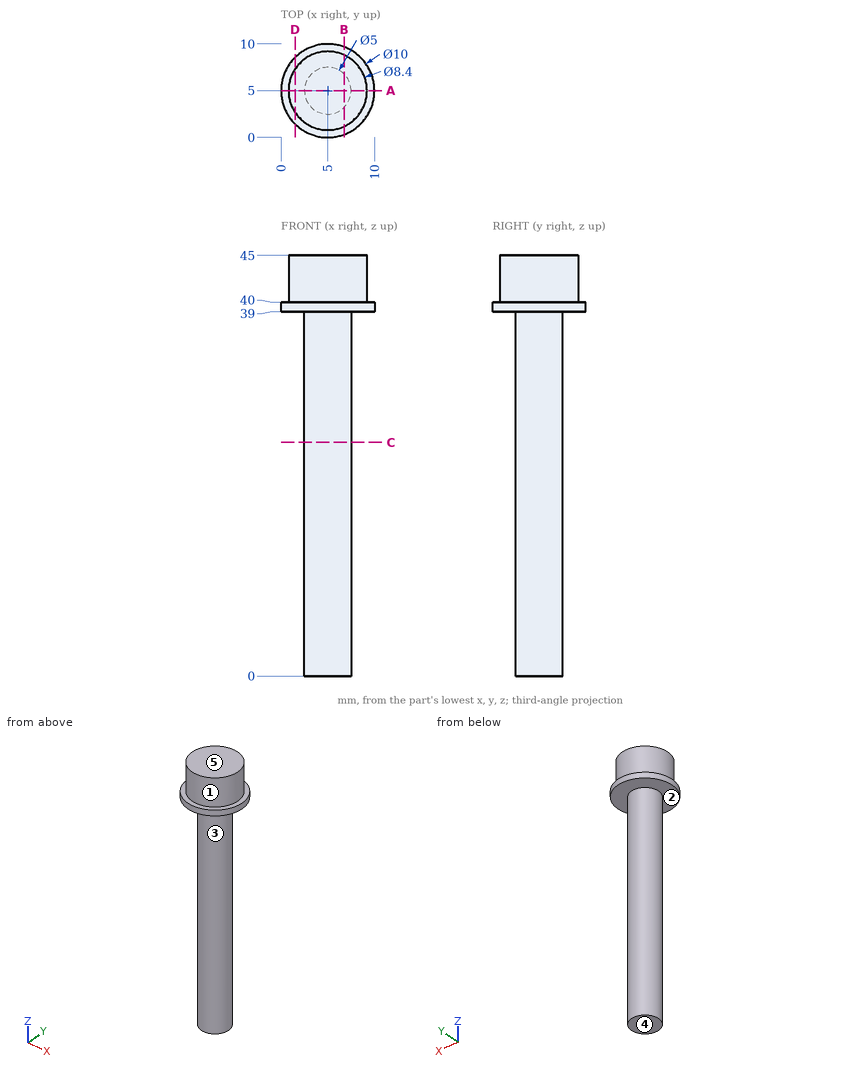
Here's the drawing with two shaded views (mm, measured from the low corner). I have some questions. A direction names the side the tool comes from. Round coordinates to 2 decimals unless told otherwise and drop trailing zeros. Order: outer loops, then holes, each group sorted by start corner. A loop starts at its lowest first (then second) coordinate and runs counter-clockwise, first axis right, second up. Notation, with made-up numbers: (15.25, 24.5) -> (51.25, 24.5) arc R23 ccw to (51.25, 35.5) -> close; hole circle Ø8 at (-36, 80.5). An arc over 180 degrees is marked (long way). Use a Markdown table: item, result. Add a question column.
(1) Suppose I cut it at A-A, the plane y = 5. Please give me the cut outline in (x, z), and give its area (3 significant figures).
(2) Suppose I cut it at C-C, the plane z = 25. Please give me the cut outline in (x, y).
(3) For pin 1 Ø1 at (x, z) = (4.5, 32) entering from +Y; pin 2 Ø1.5 at (x, z) = (3, 32) entering from -Y; pin 3 Ø5 at (x, z) = (8.5, 14.5) entering from -Y, each with a flat end and sliding along its axis, tell me the tip position at first contact or that it passes through.
(4) I need wall thicknesses on line 1 along Z through (x, y) = (8.5, 2.75); line 2 along Z through (x, y) = (9.5, 6.25); line 3 along Y through (x, z) = (3, 34). Which ranges of each line are inside material? Lowest first, please.
(5) Suppose I cut it at B-B, the plane x = 6.75. Please give me the cut outline in (y, z), and give its area (3 significant figures).
(6) Suppose I cut it at D-D, the plane x = 1.5. Please give me the cut outline in (y, z), and give its area (3 significant figures).
(7) If we mould it in two halves opening along Z, with no side actions, what happens to the marked faces 3, 4 and 5? For each: released by +Z, released by -Z, zero draft, split by the parting line, or undercut.
(8) For the marked faces 1 and 2, which set-ups out of +Z, -Z, +X, -X, +Y, -Y let a thin tool reach every point of the face, with its end or its side?
Verdict:
| question | item | result |
|---|---|---|
| 1 | outline | (0, 39) -> (2.5, 39) -> (2.5, 0) -> (7.5, 0) -> (7.5, 39) -> (10, 39) -> (10, 40) -> (9.2, 40) -> (9.2, 45) -> (0.8, 45) -> (0.8, 40) -> (0, 40) -> close |
| 1 | area | 247 mm2 |
| 2 | outline | circle Ø5 at (5, 5) |
| 3 | pin 1 | y = 7.5 |
| 3 | pin 2 | y = 2.83 |
| 3 | pin 3 | y = 2.71 |
| 4 | line 1 | 39 to 45 |
| 4 | line 2 | 39 to 40 |
| 4 | line 3 | 3.5 to 6.5 |
| 5 | outline | (0.32, 39) -> (3.21, 39) -> (3.21, 0) -> (6.79, 0) -> (6.79, 39) -> (9.68, 39) -> (9.68, 40) -> (8.82, 40) -> (8.82, 45) -> (1.18, 45) -> (1.18, 40) -> (0.32, 40) -> close |
| 5 | area | 187 mm2 |
| 6 | outline | (1.43, 39) -> (8.57, 39) -> (8.57, 40) -> (7.32, 40) -> (7.32, 45) -> (2.68, 45) -> (2.68, 40) -> (1.43, 40) -> close |
| 6 | area | 30.4 mm2 |
| 7 | face 3 | zero draft |
| 7 | face 4 | released by -Z |
| 7 | face 5 | released by +Z |
| 8 | face 1 | +Z |
| 8 | face 2 | -Z |
